```python
from build123d import *

# Parameters (mm, degrees)
F0_W           = 102
F0_H           = 124
F1_DEPTH       = 4.318
F2_W           = 102
F2_H           = 124
F2_W_2         = 90
F2_H_2         = 6
F3_DEPTH       = 8
F4_D           = 3.175
F4_CSINK_D     = 6.858
F4_CSINK_ANGLE = 90
F5_D           = 5
F7_D           = 3


with BuildPart() as f1:
    # F0 (on Top) → F1 (new body)
    with BuildSketch(Plane.XY):
        Rectangle(F0_W, F0_H)
    extrude(amount=F1_DEPTH)

    # F2 (on face) → F3 (join)
    with BuildSketch(Plane.XY.offset(4.318)):
        Rectangle(F2_W, F2_H)
        Polygon((-45, 56), (45, 56), (45, 29), (45, 0), (45, -6), (45, -33), (45, -56), (-45, -56), (-45, -33), (-45, -6), (-45, 0), (-45, 29), align=None, mode=Mode.SUBTRACT)
        with Locations((0, -3)):
            Rectangle(F2_W_2, F2_H_2)
    extrude(amount=F3_DEPTH)

    # F4 (through all)
    with Locations(Plane.XY.offset(4.318)):
        with Locations((-36, 16), (-9, 16), (9, 16), (36, 16), (9, -46), (36, -46), (-9, -46), (-36, -46)):
            CounterSinkHole(F4_D / 2, F4_CSINK_D / 2, counter_sink_angle=F4_CSINK_ANGLE)

    # F5 (through all)
    with Locations(Plane.XY.offset(4.318)):
        with Locations((-22.5, 10), (22.5, 10), (22.5, -52), (-22.5, -52)):
            Hole(F5_D / 2)

    # F7 (through all)
    with Locations(Plane.XY.offset(12.318)):
        with Locations((-48, 59), (0, 59), (48, 59), (-48, -3), (48, -3), (-48, -59), (0, -59), (48, -59), (0, -3)):
            Hole(F7_D / 2)


solid = f1.part
```
Here's how the part is built. I have some questions about the finished solid (model axes, mm). A direction names the side the tool comes from. Give positions to 0.01 mm unless a question says otherwise; leave off trailing zeros. Order: outer loops, then holes, each group sorted by start corner. A loop starts at its lowest first (then second) coordinate and runs counter-clockwise, first axis right, second up. Notation, with made-up numbers: (87, 82.25) -> (132, 82.25) arc R18 cw to (132, 91.25) -> close; hole circle Ø9 at (-32.75, 3.25). An arc over 180 degrees is marked (long way). Use CSV: the item, a comma, the result in double quotes. Start each with the question number.
Item 1: If I drill on probe 1 along Y at (x, z) = (-9, 0.8); probe 2 along Y at (x, z) = (-15, 9.5); probe 3 along X at (y, z) = (-46, 1.75), over which ranges is the centre line in solid material (lowest first)? Write a range as [from, to].
Item 2: Suppose I cut it at C-C (z = 9.25). Give the number of separate pieces and of enclosed holes in the cut face, and give its area (3 significant figures).
Item 3: On a 3-axis mill with a long thin cutter (end or side, diameter ignored), from which of +Z, -Z, +X, -X, +Y, -Y can I reach the whole of each face in a straight line? I mean faces 4 (the flat face through (1, -56, 8)), 5 (the cylindrical face through (24, 8, 2)). Say none if no direction works.
Item 4: I'm going to push a flat-ended pin straight in: P1, Ø6, axis at x = -14.5, y = -31, coming from the +Z side. Where does the tip first touch, or does it pass through?
Item 5: Thinking about a two-plate mould opening in X: for faces 1 (the cylindrical face through (49.11, -57.99, 6.07)), 2 (the flat face through (51, -1, 6)), 3 (the flat face through (-4, -4, 12.318)), which applies, pulls with the +X half, pulls with the -X half, needs draft (parallel to the pull), parting line crosses it, or undercut?
Item 6: Suppose I cut it at A-A (x = -48). List the corners of the cut face in (y, z) for me.
Item 7: Suppose I cut it at D-D (x = 36). List the corners of the cut face in (y, z) for me.
Item 8: Suppose I cut it at B-B (y = -59). List the corners of the cut face in (x, z) for me, and give its area (3 significant figures).
Answer block:
1,probe 1,"y = [-62, -47.59], [-44.41, 14.41], [17.59, 62]"
1,probe 2,"y = [-62, -56], [-6, 0], [56, 62]"
1,probe 3,"x = [-51, -37.59], [-34.41, -10.59], [-7.41, 7.41], [10.59, 34.41], [37.59, 51]"
2,separate pieces,"1"
2,enclosed holes,"11"
2,area,"3,040 mm^2"
3,face 4,"+Z"
3,face 5,"+Z, -Z"
4,P1,"stops at z = 4.32"
5,face 1,"undercut"
5,face 2,"pulls with the +X half"
5,face 3,"needs draft"
6,outline,"(-62, 0) -> (-60.5, 0) -> (-60.5, 12.32) -> (-62, 12.32) -> close; (-57.5, 0) -> (-4.5, 0) -> (-4.5, 12.32) -> (-57.5, 12.32) -> close; (-1.5, 0) -> (57.5, 0) -> (57.5, 12.32) -> (-1.5, 12.32) -> close; (60.5, 0) -> (62, 0) -> (62, 12.32) -> (60.5, 12.32) -> close"
7,outline,"(-62, 0) -> (-47.59, 0) -> (-47.59, 2.48) -> (-49.43, 4.32) -> (-56, 4.32) -> (-56, 12.32) -> (-62, 12.32) -> close; (-44.41, 0) -> (14.41, 0) -> (14.41, 2.48) -> (12.57, 4.32) -> (0, 4.32) -> (0, 12.32) -> (-6, 12.32) -> (-6, 4.32) -> (-42.57, 4.32) -> (-44.41, 2.48) -> close; (17.59, 0) -> (62, 0) -> (62, 12.32) -> (56, 12.32) -> (56, 4.32) -> (19.43, 4.32) -> (17.59, 2.48) -> close"
8,outline,"(-51, 0) -> (-49.5, 0) -> (-49.5, 12.32) -> (-51, 12.32) -> close; (-46.5, 0) -> (-1.5, 0) -> (-1.5, 12.32) -> (-46.5, 12.32) -> close; (1.5, 0) -> (46.5, 0) -> (46.5, 12.32) -> (1.5, 12.32) -> close; (49.5, 0) -> (51, 0) -> (51, 12.32) -> (49.5, 12.32) -> close"
8,area,"1,150 mm^2"
